Work out the finished part from the listing and answer in its coordinate system (mm). A direction names the side the tool comes from. Give positions to 0.01 mm unless a question says otherwise; leave off trailing zeros. Loops run counter-clockwise (first coordinate to the right, second up) from the corner with the lowest first, then second, coordinate; pieces in that order, holes last. Notation, with made-up numbers: (8, -6) -> (46, -6) arc R20 cw to (46, 8) -> close; hole circle Ø2 at (54, 86). An arc over 180 degrees is marked (long way). Answer as CSV lines item,"result". Start each with the question number.
1. Find section B-B, the plane x = 33. Give the vertices of the cut face in (y, z), and give its area (4 significant figures).
2. Find the intervals of material crossed by line 1 along Y through (x, z) = (27.5, -1.95); line 2 along X through (y, z) = (0, 0.5); line 3 along Y through (x, z) = (24, -1.3), in increasing order.
3. Find section D-D, the plane y = 15. Give the vertices of the cut face in (x, z).
4. Flat-ended cylindrical pins translate along their axes: pin 1 Ø2 at (x, z) = (49.5, -1) entering from -Y; pin 2 Ø1.5 at (x, z) = (40, -1.5) entering from -Y; pin 3 Ø1 at (x, z) = (48.5, -1.5) entering from -Y. Find the tip coordinate at first contact, or state that the pin passes through.
5. Find section C-C, the plane y = -9. Give the vertices of the cut face in (x, z), and give its area (3 significant figures).
6. A tool of negligible diameter and unlimited length cuts with its end or side. For faces 5 (the face through (39, 15, 0.5)), 6 (the face through (40, -1, -2.5)), from which of +Z, -Z, +X, -X, +Y, -Y can it reach the whole face along a straight path? Write none if from no direction.
7. Find section A-A, the plane z = -1.1. Give the vertices of the cut face in (x, y).
8. Determine the mould class of faces 1 (the face through (39, 16.5, -1)), 2 (the face through (40, 18, -2.5)), 3 (the face through (39, 20, 0)), 4 (the face through (39.4, -17.5, 0)) for opening direction Y: +Y half, -Y half, draft (parallel to the pull), parting line (faces both ways), or undercut.
from build123d import *

# Parameters (mm, degrees)
BOSS_EXTRUDE1_DEPTH     = 80
CUT_EXTRUDE1_DEPTH      = 80
SKETCH3_W               = 3
SKETCH3_H               = 3
CUT_EXTRUDE2_DEPTH      = 81
CUT_EXTRUDE2_DEPTH_BACK = 1


with BuildPart() as part:
    # Sketch1 → Boss-Extrude1 (new body)
    with BuildSketch(Plane(origin=(0, 0, 0), x_dir=(0, 0, -1), z_dir=(1, 0, 0))):
        Polygon((-2.5, -20), (2.5, -15), (2.5, 20), (-2.5, 20), align=None)
    extrude(amount=BOSS_EXTRUDE1_DEPTH)

    # Sketch2 → Cut-Extrude1 (cut)
    with BuildSketch(Plane(origin=(0, 20, 0), x_dir=(1, 0, 0), z_dir=(0, 1, 0))):
        Polygon((80, 2.5), (75, 2.5), (80, -2.5), align=None)
        Polygon((0, -2.5), (5, 2.5), (0, 2.5), align=None)
    extrude(amount=-CUT_EXTRUDE1_DEPTH, mode=Mode.SUBTRACT)

    # Sketch3 → Cut-Extrude2 (cut, two sides)
    with BuildSketch(Plane(origin=(0, 0, 0), x_dir=(0, 0, -1), z_dir=(1, 0, 0))) as cut_extrude2_sk:
        with Locations((1, 15)):
            Rectangle(SKETCH3_W, SKETCH3_H)
    extrude(amount=CUT_EXTRUDE2_DEPTH, mode=Mode.SUBTRACT)
    extrude(cut_extrude2_sk.sketch, amount=-CUT_EXTRUDE2_DEPTH_BACK, mode=Mode.SUBTRACT)


solid = part.part
Resolved:
1,outline,"(-20, 2.5) -> (-15, -2.5) -> (13.5, -2.5) -> (13.5, 0.5) -> (16.5, 0.5) -> (16.5, -2.5) -> (20, -2.5) -> (20, 2.5) -> close"
1,area,"178.5 mm^2"
2,line 1,"y = -15.55 to 13.5, 16.5 to 20"
2,line 2,"x = 2 to 78"
2,line 3,"y = -16.2 to 13.5, 16.5 to 20"
3,outline,"(0, 2.5) -> (2, 0.5) -> (78, 0.5) -> (80, 2.5) -> close"
4,pin 1,"stops at y = -17.5"
4,pin 2,"stops at y = -16.75"
4,pin 3,"stops at y = -16.5"
5,outline,"(0, 2.5) -> (5, -2.5) -> (75, -2.5) -> (80, 2.5) -> close"
5,area,"375 mm^2"
6,face 5,"-Z, +X, -X"
6,face 6,"-Z, +X, -X, +Y, -Y"
7,outline,"(3.6, -16.4) -> (76.4, -16.4) -> (76.4, 13.5) -> (3.6, 13.5) -> close; (3.6, 16.5) -> (76.4, 16.5) -> (76.4, 20) -> (3.6, 20) -> close"
8,face 1,"undercut"
8,face 2,"draft"
8,face 3,"+Y half"
8,face 4,"-Y half"
